Build history of the part. All positions in model axes, mm. Face numbers are marked on the shaded views. A direction names the side the tool comes from. Give positions to 0.01 mm unless a question says otherwise; leave off trailing zeros. Order: outer loops, then holes, each group sorted by start corner. A loop starts at its lowest first (then second) coordinate and runs counter-clockwise, first axis right, second up. Notation, with made-up numbers: M 46.25,-26 L 59.25,-26 A30 cw 59.25,6 Z; hole C -2.75,48 d3. An arc over 180 degrees is marked long. Use CSV: the item, a comma, the result in double quotes. Start each with the question number.
Item 1: Band-saw the part on B-B on y = 3. Write the cut outline in (x, z).
Item 2: Two-plate mould, pull along X, no slides. Class the marked faces 4, 5, 6 and 7: pulls with the +X half, pulls with the -X half, needs draft (parallel to the pull), parting line crosses it, or undercut.
Item 3: Wall check: line 1 along X through (y, z) = (2.45, 0); line 2 along X through (y, z) = (6.75, 0); line 3 along Z through (x, y) = (20, 2.25). Give the ranges that are in metal, low to high.
Item 4: Which spindle directions (+Z, -Z, +X, -X, +Y, -Y) get a long thin tool onto all of the face, cutting with end or side? Do the marked faces 1, 2 and 3. Say none if no direction does.
Item 5: Band-saw the part on D-D on x = 12. Write the cut outline in (y, z).
Item 6: Pin check, flat tips, straight feed: P1, Ø3, axis at x = 34.5, y = 6, coming from the +Z side; P2, Ø4.5, axis at x = 40, z = -1, coming from the +Y side; P3, Ø2, axis at x = 0.5, z = -0.5, coming from the +Y side. Stop position of each tip, or through.
Item 7: Band-saw the part on A-A on z = 0. Give the number of separate pieces and of enclosed holes in the cut face, plus the area to 3 significant figures.
Item 8: Band-saw the part on C-C on x = 20. Write the cut outline in (y, z), plus the area to 3 significant figures.
Autodesk Inventor part; units mm, degrees
ref_plane "YZ Plane" through (0, 0, 0) normal (1, 0, 0) x (0, 1, 0)
ref_plane "XZ Plane" through (0, 0, 0) normal (0, 1, 0) x (-1, 0, 0)
ref_plane "XY Plane" through (0, 0, 0) normal (0, 0, 1) x (1, 0, 0)
sketch "Sketch1" plane through (0, 0, 0) normal (0, 1, 0) x (-1, 0, 0)
  arc A0 (0, -5) -> (0, 5) centre (0, 0) ccw
  arc A1 (-40, 5) -> (-40, -5) centre (-40, 0) ccw
  line L0 (0, 5) -> (-40, 5)
  line L1 (0, -5) -> (-40, -5)
  dimension "d2" = 40
extrude "Extrusion1" add sketch "Sketch1" along normal blind 10
sketch "Sketch2" plane through (0, 10, 0) normal (0, 1, 0) x (1, 0, 0)
  point P0 (0, 0)
hole "Hole1" at (0, 10, 0) direction (0, -1, 0) diameter 3.1 end through all counterbore diameter 4 counterbore depth 5
sketch "Sketch3" plane through (0, 10, 0) normal (0, 1, 0) x (1, 0, 0)
  arc A0 (40, -5) -> (40, 5) centre (40, 0) ccw
  point P0 (0, 0)
  point P1 (20, 0)
hole "Hole2" at (40, 10, 0) at (20, 10, 0) direction (0, -1, 0) diameter 3.1 end through all counterbore diameter 4 counterbore depth 5
sketch "Sketch4" plane through (0, 0, 5) normal (0, 0, 1) x (1, 0, 0)
  line L0 (21.55, 5) -> (18.45, 5)
  line L1 (40, 10) -> (0, 10)
  line L2 (40, 0) -> (0, 0)
  line L3 (15, 10) -> (25, 10)
  line L4 (25, 10) -> (25, 0)
  line L5 (25, 0) -> (15, 0)
  line L6 (15, 0) -> (15, 10)
  point P0 (20, 5)
  dimension "d19" = 10
  dimension "d20" = 5
extrude "Extrusion2" add sketch "Sketch4" along normal blind 10
fillet "Fillet1" radius 2 14 edges at (20, 10, 15) (15, 5, 15) (20, 0, 15) (25, 5, 15) (-5, 10, 0) (20, 10, -5) (45, 10, 0) (32.5, 10, 5) (7.5, 10, 5) (-5, 0, 0) (20, 0, -5) (45, 0, 0) (32.5, 0, 5) (7.5, 0, 5)
sketch "Sketch5" plane through (0, 0, 15) normal (0, 0, 1) x (1, 0, 0)
  line L0 (21.55, 5) -> (18.45, 5)
  point P0 (0, 0)
  point P1 (20, 5)
hole "Hole3" at (20, 5, 15) direction (0, 0, -1) diameter 3.1 depth 8
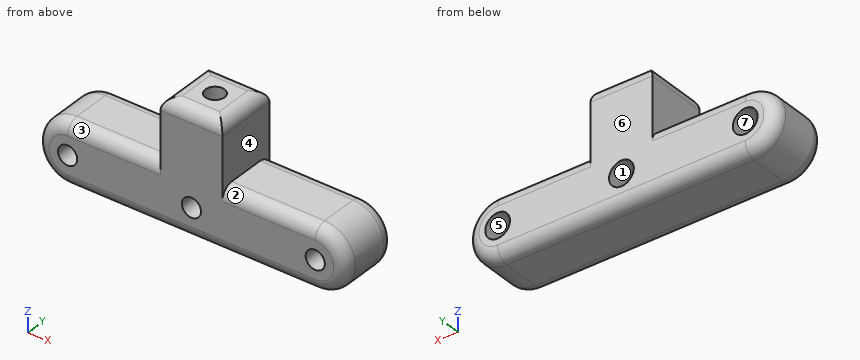
Model answer:
1,outline,"M 0,-5 L 40,-5 A5 ccw 40,5 L 25,5 L 25,13 A2 ccw 23,15 L 17,15 A2 ccw 15,13 L 15,5 L 0,5 A5 ccw Z; hole C 0,0 d3.1; hole C 20,0 d3.1; hole C 40,0 d3.1"
2,face 4,"pulls with the +X half"
2,face 5,"undercut"
2,face 6,"needs draft"
2,face 7,"undercut"
3,line 1,"x = -5 to -1.55, 1.55 to 18.45, 21.55 to 38.45, 41.55 to 45"
3,line 2,"x = -5 to -2, 2 to 18, 22 to 38, 42 to 45"
3,line 3,"z = -5 to -1.55, 1.55 to 15"
4,face 1,"+Y"
4,face 2,"+Z, +X, -Y"
4,face 3,"+Z, -X, -Y"
5,outline,"M 0,-3 A2 ccw 2,-5 L 8,-5 A2 ccw 10,-3 L 10,3 A2 ccw 8,5 L 2,5 A2 ccw 0,3 Z"
6,P1,"stops at z = 5"
6,P2,"stops at y = 10"
6,P3,"stops at y = 5"
7,separate pieces,"4"
7,enclosed holes,"0"
7,area,"390 mm^2"
8,outline,"M 0,-3 A2 ccw 2,-5 L 8,-5 A2 ccw 10,-3 L 10,-2 L 5,-2 L 5,-1.55 L 0,-1.55 Z; M 0,1.55 L 5,1.55 L 5,2 L 10,2 L 10,13 A2 ccw 8,15 L 6.55,15 L 6.55,7 L 3.45,7 L 3.45,15 L 2,15 A2 ccw 0,13 Z"
8,area,"136 mm^2"
